from build123d import *

# Parameters (mm, degrees)
F0_W           = 58
F0_H           = 6
F2_DEPTH       = 20
F3_DEPTH       = 4
F5_D           = 5.5
F5_DEPTH       = 15
F5_CSINK_D     = 11.2
F5_CSINK_ANGLE = 90
F5_TIP         = 1.6523667023
F6_R           = 5
F7_D           = 4.5
F7_DEPTH       = 15
F7_TIP         = 1.3519363928


with BuildPart() as f2:
    # F0 (on Right) → F2 (new body)
    with BuildSketch(Plane.YZ):
        with Locations((0, -3)):
            Rectangle(F0_W, F0_H)
    extrude(amount=F2_DEPTH)

    # F1 (on Right) → F3 (join)
    with BuildSketch(Plane.YZ):
        Polygon((-29, 0), (-29, -6), (29, -20), (49, -20), (49, 58), (29, 58), (29, 0), align=None)
    extrude(amount=F3_DEPTH)

    # F5
    with Locations(Plane(origin=(0, 0, -6), x_dir=(1, 0, 0), z_dir=(0, 0, -1))):
        with Locations((10, -19), (10, 19)):
            CounterSinkHole(F5_D / 2, F5_CSINK_D / 2, depth=F5_DEPTH, counter_sink_angle=F5_CSINK_ANGLE)
            with Locations((0, 0, -(F5_DEPTH + F5_TIP / 2))):  # 118° drill point
                Cone(0, F5_D / 2, F5_TIP, mode=Mode.SUBTRACT)

    # F6
    f6_edges = [f2.edges().sort_by_distance(p)[0] for p in [
        (20, -29, -3),
        (20, 29, -3),
        (2, 29, 58),
        (2, 49, 58),
        (2, 49, -20),
        (2, 29, -20),
    ]]
    fillet(f6_edges, radius=F6_R)

    # F7
    with Locations(Plane(origin=(0, 0, 0), x_dir=(0, 1, 0), z_dir=(-1, 0, 0))):
        with Locations((39, -48), (39, -19), (39, 10)):
            Hole(F7_D / 2, depth=F7_DEPTH)
            with Locations((0, 0, -(F7_DEPTH + F7_TIP / 2))):  # 118° drill point
                Cone(0, F7_D / 2, F7_TIP, mode=Mode.SUBTRACT)


solid = f2.part
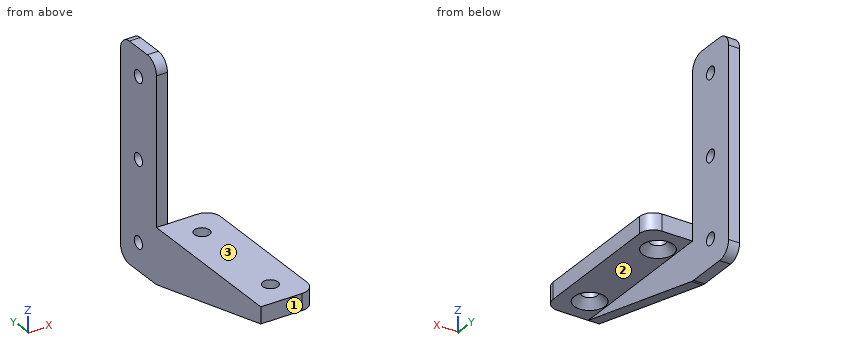
Can you work these out from the model? Positions are in its coordinate system, mm. Face numbers are marked on the shaded views. A direction names the side the tool comes from. Round coordinates to 2 decimals unless told otherwise and drop trailing zeros. Write each loop counter-clockwise with the first axis right and the second up, starting at its lowest first coordinate (ties: lowest second). Pieces come first, ordered by that corner, then holes. Notation, with made-up numbers: (-32.75, 81.5) - (19.25, 81.5) arc R35 ccw to (19.25, 118.5) - close; hole circle Ø6 at (-40, -15). An arc over 180 degrees is marked (long way). Write each question's results on one line, items separated by ' | '. Start each with the question number.
1) For pin 1 Ø6 at (x, y) = (14.5, 11) entering from +Z; pin 2 Ø6 at (y, z) = (39, -10) entering from +X; pin 3 Ø8 at (x, z) = (9.5, 12) entering from +Y; pin 4 Ø1.8 at (x, z) = (7, -3.5) entering from +Y, each with a flat end and sliding along its axis, tell me the tip position at first contact or that it passes through.
2) Which directions (+Z, -Z, +X, -X, +Y, -Y) give clear straight access to the entire face, cutting with the end or side of a thin tool? Please do the marked faces 1, 2 and 3.
3) Please list where these lines run through material, in increasing order: line 1 (Z direction, x = 1.65, y = 39); line 2 (Y direction, x = 1.6, z = 19); line 3 (X direction, y = -19, z = -1).
4) Suppose I cut it at D-D (x = 1.5). List the corners of the cut face in (y, z) for me, and give its area (3 significant figures).
5) Suppose I cut it at A-A (z = -5). List the corners of the cut face in (x, y) for me.
6) Suppose I cut it at B-B (y = 39). List the corners of the cut face in (x, z) for me, and give its area (3 significant figures).
7) Suppose I cut it at C-C (z = 19). List the corners of the cut face in (x, y) for me, and give its area (3 significant figures).
Here are the results:
1) pin 1: stops at z = 0 | pin 2: stops at x = 4 | pin 3: passes through | pin 4: stops at y = 29
2) face 1: +Z, -Z, +X, -X, -Y | face 2: -Z, +X, +Y, -Y | face 3: +Z, +X, -X, -Y
3) line 1: z = -20 to -12.25, -7.75 to 16.75, 21.25 to 45.75, 50.25 to 58 | line 2: y = 29 to 36.75, 41.25 to 49 | line 3: x = 0 to 7.25, 12.75 to 20
4) outline: (-29, -6) - (28.42, -19.86) arc R5 ccw to (29.59, -20) - (44, -20) arc R5 ccw to (49, -15) - (49, 53) arc R5 ccw to (44, 58) - (34, 58) arc R5 ccw to (29, 53) - (29, 0) - (-29, 0) - close; hole circle Ø4.5 at (39, -10); hole circle Ø4.5 at (39, 19); hole circle Ø4.5 at (39, 48) | area: 2,250 mm2
5) outline: (0, -29) - (15, -29) arc R5 ccw to (20, -24) - (20, 24) arc R5 ccw to (15, 29) - (4, 29) - (4, 49) - (0, 49) - close; hole circle Ø9.2 at (10, -19); hole circle Ø9.2 at (10, 19)
6) outline: (0, -20) - (4, -20) - (4, -12.25) - (0, -12.25) - close; (0, -7.75) - (4, -7.75) - (4, 16.75) - (0, 16.75) - close; (0, 21.25) - (4, 21.25) - (4, 45.75) - (0, 45.75) - close; (0, 50.25) - (4, 50.25) - (4, 58) - (0, 58) - close | area: 258 mm2
7) outline: (0, 29) - (4, 29) - (4, 36.75) - (0, 36.75) - close; (0, 41.25) - (4, 41.25) - (4, 49) - (0, 49) - close | area: 62.0 mm2
